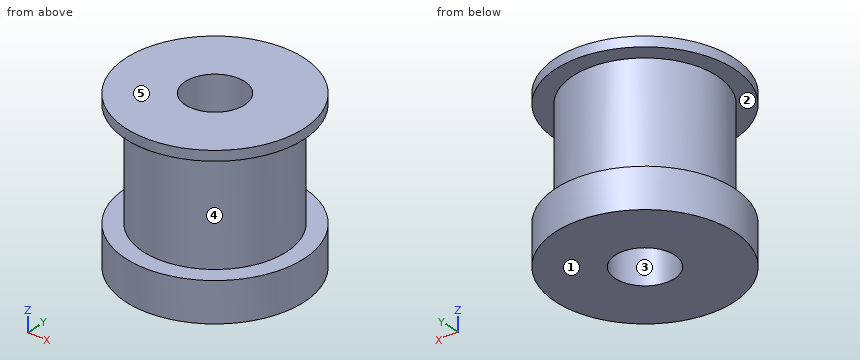
from build123d import *

# Parameters (mm, degrees)
SKETCH1_R           = 9
SKETCH1_R_2         = 3
BOSS_EXTRUDE1_DEPTH = 4
SKETCH2_R           = 7.25
SKETCH2_R_2         = 3
BOSS_EXTRUDE2_DEPTH = 11
SKETCH3_R           = 9
SKETCH3_R_2         = 3
BOSS_EXTRUDE3_DEPTH = 1
ECHELLE1_SCALE      = 2
ECHELLE2_SCALE      = 0.25


with BuildPart() as part:
    # Sketch1 → Boss-Extrude1 (new body)
    with BuildSketch(Plane.XY):
        Circle(SKETCH1_R)
        Circle(SKETCH1_R_2, mode=Mode.SUBTRACT)
    extrude(amount=BOSS_EXTRUDE1_DEPTH)

    # Sketch2 → Boss-Extrude2 (add)
    with BuildSketch(Plane.XY.offset(4)):
        Circle(SKETCH2_R)
        Circle(SKETCH2_R_2, mode=Mode.SUBTRACT)
    extrude(amount=BOSS_EXTRUDE2_DEPTH)

    # Sketch3 → Boss-Extrude3 (add)
    with BuildSketch(Plane.XY.offset(15)):
        Circle(SKETCH3_R)
        Circle(SKETCH3_R_2, mode=Mode.SUBTRACT)
    extrude(amount=BOSS_EXTRUDE3_DEPTH)


with BuildPart() as part_1:
    # Echelle1: scaled about (0, 0, 7.44086542)
    add(part.part.scale(ECHELLE1_SCALE).moved(Location((0, 0, -7.44086542))))


with BuildPart() as part_2:
    # Echelle2: scaled about (0, 0, 7.440865421)
    add(part_1.part.scale(ECHELLE2_SCALE).moved(Location((0, 0, 5.580649066))))


solid = part_2.part
Verification items for the finished model (mm, model axes). Face numbers are marked on the shaded views. A direction names the side the tool comes from. Give positions to 0.01 mm unless a question says otherwise; leave off trailing zeros. Loops run counter-clockwise (first coordinate to the right, second up) from the corner with the lowest first, then second, coordinate; pieces in that order, holes last. Notation, with made-up numbers: (-26, 11) - (11, 11) arc R17 cw to (11, 40) - close; hole circle Ø9 at (21, -24). An arc over 180 degrees is marked (long way). Write item = value, one per line. Start each with the question number.
Q1. Depth check by flat-ended pin: P1, Ø1.5, axis at x = 1.5, z = 7, coming from the -Y side. Enter the tip coordinate at first touch or a pass-through.
Q2. Thickness scan on line 1 (Z direction, x = 1.5, y = -3.75); line 2 (Y direction, x = 0, z = 9) (3 decimals); line 3 (X direction, y = 0.75, z = 6.5). Record the ranges inside material, lowest first.
Q3. Cross-section at D-D, the plane y = -3.25. Enter the section's corners in (x, z).
Q4. Cross-section at C-C, the plane z = 7. Enter the section's corners in (x, y) (3 decimals).
Q5. Tool access check on the marked faces 1 and 2. Record the directions out of +Z, -Z, +X, -X, +Y, -Y that give a thin tool (end or side, any length) a straight path to the whole face; none if there is none.
Q6. Cross-section at A-A, the plane y = 0. Enter the section's corners in (x, z) (3 decimals).
Q7. Mould release check, pull along Z, two halves, no side actions. Record for the marked faces 3, 4 and 5: released by +Z, released by -Z, zero draft, split by the parting line, or undercut.
Answer key:
q1.P1 = -3.55
q2.line_1 = 3.72 to 5.72, 11.22 to 11.72
q2.line_2 = -3.625 to -1.5, 1.5 to 3.625
q2.line_3 = -3.55 to -1.3, 1.3 to 3.55
q3.outline = (-3.11, 3.72) - (3.11, 3.72) - (3.11, 5.72) - (1.61, 5.72) - (1.61, 11.22) - (3.11, 11.22) - (3.11, 11.72) - (-3.11, 11.72) - (-3.11, 11.22) - (-1.61, 11.22) - (-1.61, 5.72) - (-3.11, 5.72) - close
q4.outline = circle Ø7.25 at (0, 0); hole circle Ø3 at (0, 0)
q5.face_1 = -Z, +X, -X, +Y, -Y
q5.face_2 = none
q6.outline = (-4.5, 3.72) - (-1.5, 3.72) - (-1.5, 11.72) - (-4.5, 11.72) - (-4.5, 11.22) - (-3.625, 11.22) - (-3.625, 5.72) - (-4.5, 5.72) - close; (1.5, 3.72) - (4.5, 3.72) - (4.5, 5.72) - (3.625, 5.72) - (3.625, 11.22) - (4.5, 11.22) - (4.5, 11.72) - (1.5, 11.72) - close
q7.face_3 = zero draft
q7.face_4 = undercut
q7.face_5 = released by +Z
